Input: part model. Units: mm. Frame: model coordinates. A direction names the side the tool comes from. Give positions to 0.01 mm unless a question says otherwise; leave off trailing zeros. Write each loop counter-clockwise with the first axis right and the second up, starting at its lowest first coordinate (ties: lowest second). Pieces come first, ordered by that corner, then holes. Notation, with made-up numbers: (58, 42.25) - (94, 42.25) arc R28 ccw to (94, 67.25) - close; hole circle Ø7 at (16, -2.5). An arc over 180 degrees is marked (long way). Use a Markdown table: item, result. Add a question column.
1. Pin query (flat end, axial travel): pin 1 (1.5 mm diameter, centred on x = 23.5, z = 2, fed in from -Y); pin 2 (3 mm diameter, centred on x = -5, z = 4.5, fed in from -Y). Return the tip coordinate at first contact, or that it passes through.
2. Section query A-A, the plane x = 14. Return loops of the section in (y, z), plus the area to 3 significant figures.
3. Mould query, pull axis Y, two halves, no side actions, for faces 4 (the cylindrical face through (-2.38, -10.74, 3.45)), 5 (the cylindrical face through (-44.426, 5.857, 3.451)), 6 (the flat face through (3.47, 14.96, 3.45)), 7 (the cylindrical face through (37.41, -15.14, 3.45)). Classes: released by +Y, released by -Y, zero draft, split by the parting line, or undercut.
4. Section query D-D, the plane y = -15. Return loops of the section in (x, z).
5. Section query B-B, the plane y = -7.5. Return loops of the section in (x, z), plus the area to 3 significant figures.
6. Section query C-C, the plane y = -20. Return loops of the section in (x, z), plus the area to 3 significant figures.
7. Set-up query: faces 1 (the flat face through (-3.447, 14.9, 3.451)), 2 (the flat face through (-11, 5, 7)), 3 (the flat face through (0.73, -14.96, 3.45)). Return all of +Z, -Z, +X, -X, +Y, -Y with unobstructed straight access to the full face (end or side cutting, diameter ignored); none if empty.
8. Material intervals for probe 1 along X at (y, z) = (0.5, 6.5); probe 2 along X at (y, z) = (-4, 3.5); probe 3 along X at (y, z) = (-15.5, 4.5), sorted ascending.
```python
from build123d import *

# Parameters (mm, degrees)
F0_R     = 11
F1_DEPTH = 7


# Not quite as in the source:
# - a feature names something its author has since deleted; it is built from what else it names


with BuildPart() as f1:
    # F0 (on Top) → F1 (new body)
    with BuildSketch(Plane.XY):
        with BuildLine():
            ThreePointArc((8.2670150988, 10.0327693762), (6.6928166447, 10.8047053779), (5.3005300857, 11.87031511))
            ThreePointArc((5.3005300857, 11.87031511), (3.9954022113, 12.3708027698), (2.6440826014, 12.7282688217))
            ThreePointArc((2.6440826014, 12.7282688217), (0, 13), (-2.6440826014, 12.7282688217))
            ThreePointArc((-2.6440826014, 12.7282688217), (-3.9954022113, 12.3708027698), (-5.3005300857, 11.87031511))
            ThreePointArc((-5.3005300857, 11.87031511), (-6.6928166447, 10.8047053779), (-8.2670150988, 10.0327693762))
            ThreePointArc((-8.2670150988, 10.0327693762), (-11.5023304401, 6.0577549014), (-12.9498157312, 1.1411715589))
            ThreePointArc((-12.9498157312, 1.1411715589), (-10.91097159, -7.0675808423), (-4.2533323097, -12.2845091177))
            ThreePointArc((-4.2533323097, -12.2845091177), (-2.8648005364, -12.5913760507), (-1.4801854989, -12.9154578273))
            ThreePointArc((-1.4801854989, -12.9154578273), (0, -13), (1.4801854989, -12.9154578273))
            ThreePointArc((1.4801854989, -12.9154578273), (2.8648005364, -12.5913760507), (4.2533323097, -12.2845091177))
            ThreePointArc((4.2533323097, -12.2845091177), (10.5899320117, -7.5401153829), (13, 0))
            ThreePointArc((13, 0), (12.9870943447, 0.5791204378), (12.9484030029, 1.1570910404))
            ThreePointArc((12.9484030029, 1.1570910404), (11.4986046018, 6.0648241699), (8.2670150988, 10.0327693762))
        make_face()
        Circle(F0_R, mode=Mode.SUBTRACT)
        with BuildLine():
            ThreePointArc((2.6440826014, 12.7282688217), (3.9954022113, 12.3708027698), (5.3005300857, 11.87031511))
            Line((5.3005300857, 11.87031511), (4.2731994612, 17.1326149936))
            Line((4.2731994612, 17.1326149936), (2.6440826014, 12.7282688217))
        make_face()
        with BuildLine():
            ThreePointArc((8.2670150988, 10.0327693762), (6.8457077183, 11.0515286651), (5.3005300857, 11.87031511))
            ThreePointArc((5.3005300857, 11.87031511), (6.6928166447, 10.8047053779), (8.2670150988, 10.0327693762))
        make_face()
        with BuildLine():
            ThreePointArc((20.2180479346, 17.345385846), (16.0230615621, 10.7791515778), (8.2670150988, 10.0327693762))
            ThreePointArc((8.2670150988, 10.0327693762), (11.4986046018, 6.0648241699), (12.9484030029, 1.1570910404))
            ThreePointArc((12.9484030029, 1.1570910404), (12.9870943447, 0.5791204378), (13, 0))
            ThreePointArc((13, 0), (10.5899320117, -7.5401153829), (4.2533323097, -12.2845091177))
            ThreePointArc((4.2533323097, -12.2845091177), (17.1543822867, -10.2782846696), (30.1999320971, -9.7532540138))
            ThreePointArc((30.1999320971, -9.7532540138), (37.492259841, -15.2381838585), (41.3699261844, -23.4980992973))
            ThreePointArc((41.3699261844, -23.4980992973), (44.5988308489, 5.4669473875), (21.2553682043, 22.9163744996))
            ThreePointArc((21.2553682043, 22.9163744996), (20.8964882238, 20.1011290455), (20.2180479346, 17.345385846))
        make_face()
        with BuildLine():
            ThreePointArc((34.9047439829, 2.1361683247), (24.3947690942, -8.8529114999), (12.9484030029, 1.1570910404))
            ThreePointArc((12.9484030029, 1.1570910404), (23.4147188717, 13.1252481492), (34.9047439829, 2.1361683247))
        make_face(mode=Mode.SUBTRACT)
        with BuildLine():
            ThreePointArc((-5.3005300857, 11.87031511), (-3.9954022113, 12.3708027698), (-2.6440826014, 12.7282688217))
            Line((-2.6440826014, 12.7282688217), (-4.2731994612, 17.1326149936))
            Line((-4.2731994612, 17.1326149936), (-5.3005300857, 11.87031511))
        make_face()
        with BuildLine():
            ThreePointArc((-8.2670150988, 10.0327693762), (-6.6928166447, 10.8047053779), (-5.3005300857, 11.87031511))
            ThreePointArc((-5.3005300857, 11.87031511), (-6.8457077183, 11.0515286651), (-8.2670150988, 10.0327693762))
        make_face()
        with BuildLine():
            ThreePointArc((-12.9498157312, 1.1411715589), (-11.5023304401, 6.0577549014), (-8.2670150988, 10.0327693762))
            ThreePointArc((-8.2670150988, 10.0327693762), (-16.0230615621, 10.7791515778), (-20.2180479346, 17.345385846))
            ThreePointArc((-20.2180479346, 17.345385846), (-20.8964882238, 20.1011290455), (-21.2553682043, 22.9163744996))
            ThreePointArc((-21.2553682043, 22.9163744996), (-44.5988308489, 5.4669473875), (-41.3699261844, -23.4980992973))
            ThreePointArc((-41.3699261844, -23.4980992973), (-37.492259841, -15.2381838585), (-30.1999320971, -9.7532540138))
            ThreePointArc((-30.1999320971, -9.7532540138), (-17.1543822867, -10.2782846696), (-4.2533323097, -12.2845091177))
            ThreePointArc((-4.2533323097, -12.2845091177), (-10.91097159, -7.0675808423), (-12.9498157312, 1.1411715589))
        make_face()
        with BuildLine():
            ThreePointArc((-12.9073521155, 2.1067783052), (-12.917973147, 1.6235083115), (-12.9498157312, 1.1411715589))
            ThreePointArc((-12.9498157312, 1.1411715589), (-34.896731084, 2.5900482989), (-12.9073521155, 2.1067783052))
        make_face(mode=Mode.SUBTRACT)
        with BuildLine():
            Line((0, -16.953125596), (1.4801854989, -12.9154578273))
            ThreePointArc((1.4801854989, -12.9154578273), (0, -13), (-1.4801854989, -12.9154578273))
            Line((-1.4801854989, -12.9154578273), (0, -16.953125596))
        make_face()
    extrude(amount=F1_DEPTH)


solid = f1.part
```
Result sheet:
| question | item | result |
|---|---|---|
| 1 | pin 1 | stops at y = -9.87 |
| 1 | pin 2 | stops at y = -12.45 |
| 2 | outline | (-10.63, 0) - (-2.65, 0) - (-2.65, 7) - (-10.63, 7) - close; (6.92, 0) - (9.87, 0) - (9.87, 7) - (6.92, 7) - close |
| 2 | area | 76.5 mm² |
| 3 | face 4 | undercut |
| 3 | face 5 | split by the parting line |
| 3 | face 6 | released by +Y |
| 3 | face 7 | released by -Y |
| 4 | outline | (-45.66, 0) - (-37.3, 0) - (-37.3, 7) - (-45.66, 7) - close; (-0.72, 0) - (0.72, 0) - (0.72, 7) - (-0.72, 7) - close; (37.3, 0) - (45.66, 0) - (45.66, 7) - (37.3, 7) - close |
| 5 | outline | (-46.99, 0) - (-29.27, 0) - (-29.27, 7) - (-46.99, 7) - close; (-18.55, 0) - (-8.05, 0) - (-8.05, 7) - (-18.55, 7) - close; (8.05, 0) - (18.6, 0) - (18.6, 7) - (8.05, 7) - close; (29.21, 0) - (46.99, 0) - (46.99, 7) - (29.21, 7) - close |
| 5 | area | 396 mm² |
| 6 | outline | (-43.57, 0) - (-40.32, 0) - (-40.32, 7) - (-43.57, 7) - close; (40.32, 0) - (43.57, 0) - (43.57, 7) - (40.32, 7) - close |
| 6 | area | 45.5 mm² |
| 7 | face 1 | +Z, -Z, +Y |
| 7 | face 2 | +Z, +X, -X, +Y, -Y |
| 7 | face 3 | +Z, -Z, -Y |
| 8 | probe 1 | x = -46.24 to -34.79, -13.03 to -10.99, 10.99 to 13.03, 34.78 to 46.24 |
| 8 | probe 2 | x = -46.93 to -33.06, -14.76 to -10.25, 10.25 to 14.78, 33.03 to 46.93 |
| 8 | probe 3 | x = -45.5 to -37.7, -0.53 to 0.53, 37.7 to 45.5 |
